Source: CAD feature listing. Evaluate the final solid. Frame: model axes, mm. Round coordinates to 2 decimals unless told otherwise and drop trailing zeros. Write each loop counter-clockwise with the first axis right and the second up, starting at its lowest first coordinate (ties: lowest second). Pieces come first, ordered by that corner, then holes.
from build123d import *

# Parameters (mm, degrees)
F0_W             = 120
F0_H             = 150
F1_DEPTH         = 8
F2_R             = 2
F3_DEPTH         = 8
F3_COPIES_COUNT  = 3
F3_COPIES_PITCH  = 36
F3_COPIES2_COUNT = 2
F3_COPIES2_PITCH = 103.247276
F4_R             = 3.25
F4_W             = 120
F4_H             = 16
F4_R_2           = 2.5
F5_DEPTH         = 8


# Not quite as in the source:
# - a pattern or mirror of a feature is missing from the dataset's text; its kind, count and spacing are read off the source's solid


with BuildPart() as f1:
    # F0 (on Top) → F1 (new body)
    with BuildSketch(Plane.XY):
        Rectangle(F0_W, F0_H)
    extrude(amount=F1_DEPTH)

    # F2 (on face) → F3 (cut, through all)
    with BuildSketch(Plane.XY.offset(8)):
        with Locations((-54, 54)):
            Circle(F2_R)
        with Locations((-18, 54)):
            Circle(F2_R)
        with Locations((-18, 20)):
            Circle(F2_R)
        with Locations((-54, 20)):
            Circle(F2_R)
    f3 = extrude(amount=-F3_DEPTH, mode=Mode.SUBTRACT)

    # F3_copies: F3 ×3
    with Locations(*[(i * F3_COPIES_PITCH, 0, 0) for i in range(1, F3_COPIES_COUNT)]):
        add(f3, mode=Mode.SUBTRACT)

    # F3_copies1: F3 across plane
    add(f3.mirror(Plane(origin=(0, 0, 0), x_dir=(0, 0, -1), z_dir=(0, -1, 0))), mode=Mode.SUBTRACT)

    # F3_copies2: F3 ×2
    with Locations(*[Vector(0.6973549598, -0.7167259309, 0) * (i * F3_COPIES2_PITCH) for i in range(1, F3_COPIES2_COUNT)]):
        add(f3, mode=Mode.SUBTRACT)

    # F4 (on face) → F5 (cut, through all)
    with BuildSketch(Plane.XY.offset(8)):
        with Locations((-14, -4)):
            Circle(F4_R)
        with Locations((14, -4)):
            Circle(F4_R)
        with Locations((0, -67)):
            Rectangle(F4_W, F4_H)
        with Locations((38, -29)):
            Circle(F4_R_2)
        with Locations((38, 45)):
            Circle(F4_R_2)
        with Locations((-38, 45)):
            Circle(F4_R_2)
        with Locations((-38, -29)):
            Circle(F4_R_2)
    extrude(amount=-F5_DEPTH, mode=Mode.SUBTRACT)


solid = f1.part
1) Contact query for a flat-ended pin moving along its axis: P1, Ø2.5, axis at x = 54, y = -20, coming from the +Z side. Output: stop coordinate, or through.
Taken from the geometry:
P1: passes through
2) Material intervals for line 1 (Y direction, x = 54, z = 4); line 2 (Y direction, x = 38, z = 3.75); line 3 (X direction, y = -54, z = 2.5), sorted ascending.
Taken from the geometry:
line 1: y = -59 to -56, -52 to -22, -18 to 18, 22 to 52, 56 to 75
line 2: y = -59 to -31.5, -26.5 to 42.5, 47.5 to 75
line 3: x = -60 to -56, -52 to -20, -16 to 16, 20 to 52, 56 to 60
3) Section query D-D on x = -14. Return the cut outline in (y, z).
Taken from the geometry:
outline: (-59, 0) - (-7.25, 0) - (-7.25, 8) - (-59, 8) - close; (-0.75, 0) - (75, 0) - (75, 8) - (-0.75, 8) - close
4) Section query C-C on y = 45. Return the cut outline in (x, z), then the cut area to 3 significant figures.
Taken from the geometry:
outline: (-60, 0) - (-40.5, 0) - (-40.5, 8) - (-60, 8) - close; (-35.5, 0) - (35.5, 0) - (35.5, 8) - (-35.5, 8) - close; (40.5, 0) - (60, 0) - (60, 8) - (40.5, 8) - close
area: 880 mm2
5) Pull-direction query (X, two-part tool) for faces 1 (the face through (18, -52, 4)), 2 (the face through (-1, 9, 0)), 3 (the face through (-60, 7, 4)); classes: released by +X, released by -X, zero draft, split by the parting line, or undercut.
Taken from the geometry:
face 1: undercut
face 2: zero draft
face 3: released by -X
6) Section query B-B on x = -54. Return the cut outline in (y, z).
Taken from the geometry:
outline: (-59, 0) - (-56, 0) - (-56, 8) - (-59, 8) - close; (-52, 0) - (-22, 0) - (-22, 8) - (-52, 8) - close; (-18, 0) - (18, 0) - (18, 8) - (-18, 8) - close; (22, 0) - (52, 0) - (52, 8) - (22, 8) - close; (56, 0) - (75, 0) - (75, 8) - (56, 8) - close
7) Section query A-A on z = 6.25. State how many separate pieces and enclosed holes the cut face has, then the cut area to 3 significant figures.
Taken from the geometry:
separate pieces: 1
enclosed holes: 22
area: 15,700 mm2
